from build123d import *

# Parameters (mm, degrees)
F0_W      = 20
F0_H      = 20
F1_DEPTH  = 20
F5_R      = 2
F8_DEPTH  = 0.9
F2_R      = 2
F9_DEPTH  = 0.9
F4_R      = 2
F10_DEPTH = 0.9
F7_R      = 2
F11_DEPTH = 0.9
F12_DEPTH = 0.9
F3_R      = 2
F13_DEPTH = 0.9
F14_R     = 1.99999


# Not quite as in the source:
# - a fillet or chamfer is up to 0.001 mm smaller than in the source, because OpenCascade refuses the exact size


with BuildPart() as f1:
    # F0 (on Top) → F1 (new body)
    with BuildSketch(Plane.XY):
        with Locations((10, 10)):
            Rectangle(F0_W, F0_H)
    extrude(amount=F1_DEPTH)

    # F5 (on face) → F8 (cut)
    with BuildSketch(Plane(origin=(0, 0, 0), x_dir=(0, -1, 0), z_dir=(-1, 0, 0))):
        with Locations((-16, 16)):
            Circle(F5_R)
        with Locations((-10, 10)):
            Circle(F5_R)
        with Locations((-4, 16)):
            Circle(F5_R)
        with Locations((-4, 4)):
            Circle(F5_R)
        with Locations((-16, 4)):
            Circle(F5_R)
    extrude(amount=-F8_DEPTH, mode=Mode.SUBTRACT)

    # F2 (on face) → F9 (cut)
    with BuildSketch(Plane.XY.offset(20)):
        with Locations((10, 10)):
            Circle(F2_R)
    extrude(amount=-F9_DEPTH, mode=Mode.SUBTRACT)

    # F4 (on face) → F10 (cut)
    with BuildSketch(Plane.YZ.offset(20)):
        with Locations((13.3333333333, 6.6666666667)):
            Circle(F4_R)
        with Locations((6.6666666667, 13.3333333333)):
            Circle(F4_R)
    extrude(amount=-F10_DEPTH, mode=Mode.SUBTRACT)

    # F7 (on face) → F11 (cut)
    with BuildSketch(Plane(origin=(0, 20, 0), x_dir=(-1, 0, 0), z_dir=(0, 1, 0))):
        with Locations((-3.9495522901, 16.0504477099)):
            Circle(F7_R)
        with Locations((-3.9495522901, 3.9495522901)):
            Circle(F7_R)
        with Locations((-16.0504477099, 3.9495522901)):
            Circle(F7_R)
        with Locations((-16.0504477099, 16.0504477099)):
            Circle(F7_R)
    extrude(amount=-F11_DEPTH, mode=Mode.SUBTRACT)

    # F6 (on face) → F12 (cut)
    with BuildSketch(Plane.XZ):
        with BuildLine():
            Line((15.2621462241, 4.7378537759), (13.8479326617, 6.1520673383))
            ThreePointArc((13.8479326617, 6.1520673383), (13.8479326617, 3.3236402136), (16.6763597864, 3.3236402136))
            Line((16.6763597864, 3.3236402136), (15.2621462241, 4.7378537759))
        make_face()
        with BuildLine():
            ThreePointArc((17.2621462241, 4.7378537759), (16.0275130888, 6.585612841), (13.8479326617, 6.1520673383))
            Line((13.8479326617, 6.1520673383), (15.2621462241, 4.7378537759))
            Line((15.2621462241, 4.7378537759), (16.6763597864, 3.3236402136))
            ThreePointArc((16.6763597864, 3.3236402136), (17.1099052891, 3.9724869112), (17.2621462241, 4.7378537759))
        make_face()
        with BuildLine():
            ThreePointArc((11.3126059573, 10.6873940427), (10.077972822, 12.5351531078), (7.8983923949, 12.1016076051))
            Line((7.8983923949, 12.1016076051), (9.3126059573, 10.6873940427))
            Line((9.3126059573, 10.6873940427), (10.7268195196, 9.2731804804))
            ThreePointArc((10.7268195196, 9.2731804804), (11.1603650223, 9.922027178), (11.3126059573, 10.6873940427))
        make_face()
        with BuildLine():
            Line((9.3126059573, 10.6873940427), (7.8983923949, 12.1016076051))
            ThreePointArc((7.8983923949, 12.1016076051), (7.8983923949, 9.2731804804), (10.7268195196, 9.2731804804))
            Line((10.7268195196, 9.2731804804), (9.3126059573, 10.6873940427))
        make_face()
        with BuildLine():
            ThreePointArc((5.475499908, 14.524500092), (5.9090454106, 15.1733467897), (6.0612863456, 15.9387136544))
            ThreePointArc((6.0612863456, 15.9387136544), (4.8266532103, 17.7864727194), (2.6470727832, 17.3529272168))
            Line((2.6470727832, 17.3529272168), (4.0612863456, 15.9387136544))
            Line((4.0612863456, 15.9387136544), (5.475499908, 14.524500092))
        make_face()
        with BuildLine():
            Line((4.0612863456, 15.9387136544), (2.6470727832, 17.3529272168))
            ThreePointArc((2.6470727832, 17.3529272168), (2.6470727832, 14.524500092), (5.475499908, 14.524500092))
            Line((5.475499908, 14.524500092), (4.0612863456, 15.9387136544))
        make_face()
    extrude(amount=-F12_DEPTH, mode=Mode.SUBTRACT)

    # F3 (on face) → F13 (cut)
    with BuildSketch(Plane(origin=(0, 0, 0), x_dir=(1, 0, 0), z_dir=(0, 0, -1))):
        with Locations((15.949013711, -4.050986289)):
            Circle(F3_R)
        with Locations((15.949013711, -10)):
            Circle(F3_R)
        with Locations((15.949013711, -15.949013711)):
            Circle(F3_R)
        with Locations((4.050986289, -4.050986289)):
            Circle(F3_R)
        with Locations((4.050986289, -10)):
            Circle(F3_R)
        with Locations((4.050986289, -15.949013711)):
            Circle(F3_R)
    extrude(amount=-F13_DEPTH, mode=Mode.SUBTRACT)

    # F14 (radius 2 in the source; OpenCascade refuses exactly that, so slightly less here)
    f14_edges = [f1.edges().sort_by_distance(p)[0] for p in [
        (20, 10, 0),
        (10, 20, 0),
        (0, 20, 10),
        (0, 10, 20),
        (10, 20, 20),
        (20, 10, 20),
        (20, 0, 10),
        (10, 0, 20),
        (20, 20, 10),
        (0, 10, 0),
        (0, 0, 10),
        (10, 0, 0),
    ]]
    fillet(f14_edges, radius=F14_R)


solid = f1.part
Work out the finished part from the listing and answer in its coordinate system (mm). A direction names the side the tool comes from. Round coordinates to 2 decimals unless told otherwise and drop trailing zeros. Write each loop counter-clockwise with the first axis right and the second up, starting at its lowest first coordinate (ties: lowest second). Pieces come first, ordered by that corner, then holes.
1) A cutting plane is placed at C-C (z = 13). Give the vertices of the cut face in (x, y).
2) The mould has two halves that part along Z. Classify faces 6 (the flat face through (0.9, 4, 16)), 7 (the cylindrical face through (19.4, 10.11, 19.43)), 8 (the flat face through (4, 16, 0.9)): pulls with the +Z half, pulls with the -Z half, needs draft (parallel to the pull), parting line crosses it, or undercut.
3) Given pin 1 Ø12 at (x, z) = (14.5, 8) entering from -Y; pin 2 Ø1.2 at (x, y) = (4.5, 9.5) entering from -Z; pin 3 Ø3.5 at (x, z) = (16.05, 16.05) entering from +Y; pin 4 Ø2.5 at (y, z) = (16, 16) entering from -X, each flat-ended and moving along its own axis, determine where each tip first touches the part or whether it passes through.
4) A cutting plane is placed at A-A (y = 10). Give the vertices of the cut face in (x, z), plus the area to 3 significant figures.
5) A cutting plane is placed at B-B (x = 10). Give the vertices of the cut face in (y, z).
6) A tool of negligible diameter and unlimited length cuts with its end or side. For faces 1 (the cylindrical face through (0.444, 16.26, 17.983)), 2 (the flat face through (10, 10, 0)), 3 (the flat face through (16, 4, 0.9)), 4 (the cylindrical face through (18.05, 19.56, 4.04)), 5 (the flat face through (19.1, 13, 7)), from which of +Z, -Z, +X, -X, +Y, -Y can it reach the whole face along a straight path? Write none if from no direction.
7) Straight lines are drawn through the part: line 1 (Z direction, x = 0.65, y = 16); line 2 (Z direction, x = 3.5, y = 17.5); line 3 (Y direction, x = 5, z = 2.5). For each, find the intervals that lie inside material, in ascending order.
Completed:
1. outline: (0, 2) arc R2 ccw to (2, 0) - (18, 0) arc R2 ccw to (20, 2) - (20, 4.69) - (19.1, 4.69) - (19.1, 8.64) - (20, 8.64) - (20, 18) arc R2 ccw to (18, 20) - (2, 20) arc R2 ccw to (0, 18) - close
2. face 6: undercut
2. face 7: pulls with the +Z half
2. face 8: pulls with the -Z half
3. pin 1: stops at y = 0
3. pin 2: stops at z = 0.9
3. pin 3: stops at y = 19.1
3. pin 4: stops at x = 0.9
4. outline: (0, 2) arc R2 ccw to (2, 0) - (2.05, 0) - (2.05, 0.9) - (6.05, 0.9) - (6.05, 0) - (13.95, 0) - (13.95, 0.9) - (17.95, 0.9) - (17.95, 0) - (18, 0) arc R2 ccw to (20, 2) - (20, 18) arc R2 ccw to (18, 20) - (12, 20) - (12, 19.1) - (8, 19.1) - (8, 20) - (2, 20) arc R2 ccw to (0, 18) - (0, 12) - (0.9, 12) - (0.9, 8) - (0, 8) - close
4. area: 382 mm2
5. outline: (0, 2) arc R2 ccw to (2, 0) - (18, 0) arc R2 ccw to (20, 2) - (20, 18) arc R2 ccw to (18, 20) - (12, 20) - (12, 19.1) - (8, 19.1) - (8, 20) - (2, 20) arc R2 ccw to (0, 18) - (0, 12.57) - (0.9, 12.57) - (0.9, 8.81) - (0, 8.81) - close
6. face 1: -X
6. face 2: -Z, +X, -X, +Y, -Y
6. face 3: -Z
6. face 4: +Y
6. face 5: +X
7. line 1: z = 0.52 to 2, 6 to 14, 18 to 19.48
7. line 2: z = 0.9 to 20
7. line 3: y = 0 to 19.1
